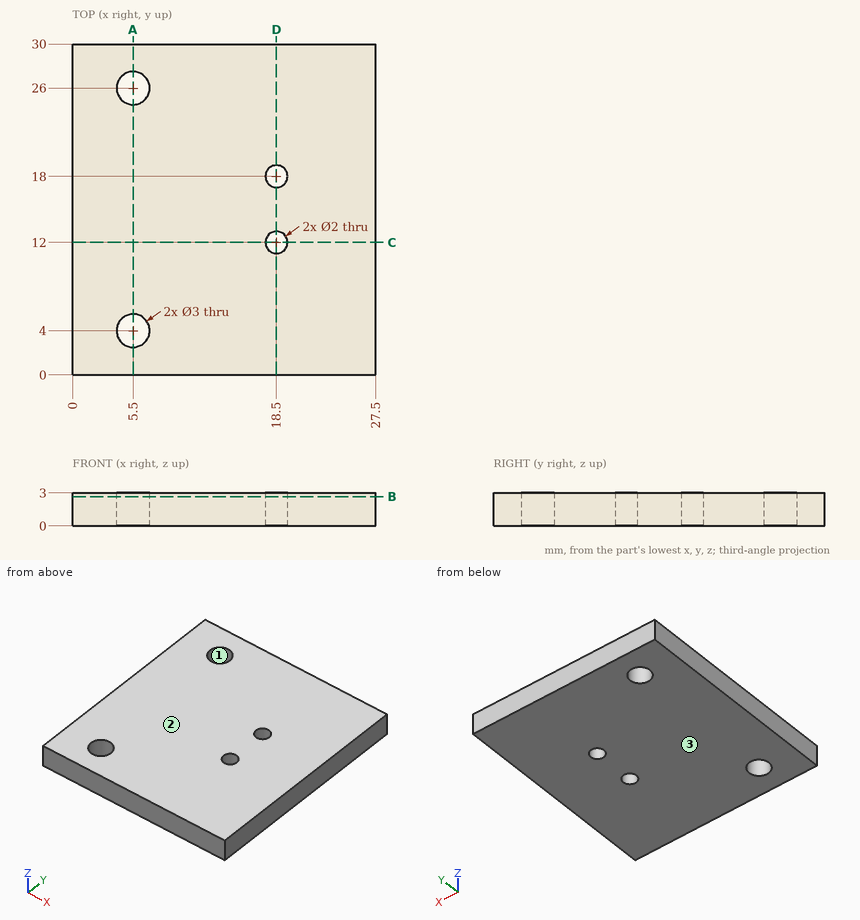
Drawing for the job (mm, zero at the part's lowest x, y, z). Round coordinates to 2 decimals unless told otherwise and drop trailing zeros. Write each loop counter-clockwise with the first axis right and the second up, starting at its lowest first coordinate (ties: lowest second). Pieces come first, ordered by that corner, then holes. Notation, with made-up numbers: M 11.25,10.5 L 23.25,10.5 A25 ccw 23.25,26.5 Z; hole C 25.5,28 d7. An arc over 180 degrees is marked long. Answer in a Markdown table with one row per item.
1. Saw through at C-C (y = 12). List the corners of the cut face in (x, z), and give its area (3 significant figures).
Geometry check:
| item | result |
|---|---|
| outline | M 0,0 L 17.5,0 L 17.5,3 L 0,3 Z; M 19.5,0 L 27.5,0 L 27.5,3 L 19.5,3 Z |
| area | 76.5 mm2 |
2. Saw through at B-B (z = 2.65). List the corners of the cut face in (x, y).
Geometry check:
| item | result |
|---|---|
| outline | M 0,0 L 27.5,0 L 27.5,30 L 0,30 Z; hole C 5.5,4 d3; hole C 5.5,26 d3; hole C 18.5,12 d2; hole C 18.5,18 d2 |
3. Mould opens along Z. For the marked faces 1, 2 and 3 say: +Z half, -Z half, draft (parallel to the pull), parting line (faces both ways), or undercut.
Geometry check:
| item | result |
|---|---|
| face 1 | draft |
| face 2 | +Z half |
| face 3 | -Z half |
4. Probe L1, parallel to Y at x = 18.5, z = 2.05; L2, parallel to Y at x = 5.5, z = 1.4; L3, parallel to X at y = 26, z = 0.7. List the from-to ranges inside material, lowest first. Write a range as [from, to].
Geometry check:
| item | result |
|---|---|
| L1 | [0, 11], [13, 17], [19, 30] |
| L2 | [0, 2.5], [5.5, 24.5], [27.5, 30] |
| L3 | [0, 4], [7, 27.5] |
5. Saw through at A-A (x = 5.5). List the corners of the cut face in (y, z).
Geometry check:
| item | result |
|---|---|
| outline | M 0,0 L 2.5,0 L 2.5,3 L 0,3 Z; M 5.5,0 L 24.5,0 L 24.5,3 L 5.5,3 Z; M 27.5,0 L 30,0 L 30,3 L 27.5,3 Z |
6. Saw through at D-D (x = 18.5). List the corners of the cut face in (y, z).
Geometry check:
| item | result |
|---|---|
| outline | M 0,0 L 11,0 L 11,3 L 0,3 Z; M 13,0 L 17,0 L 17,3 L 13,3 Z; M 19,0 L 30,0 L 30,3 L 19,3 Z |
